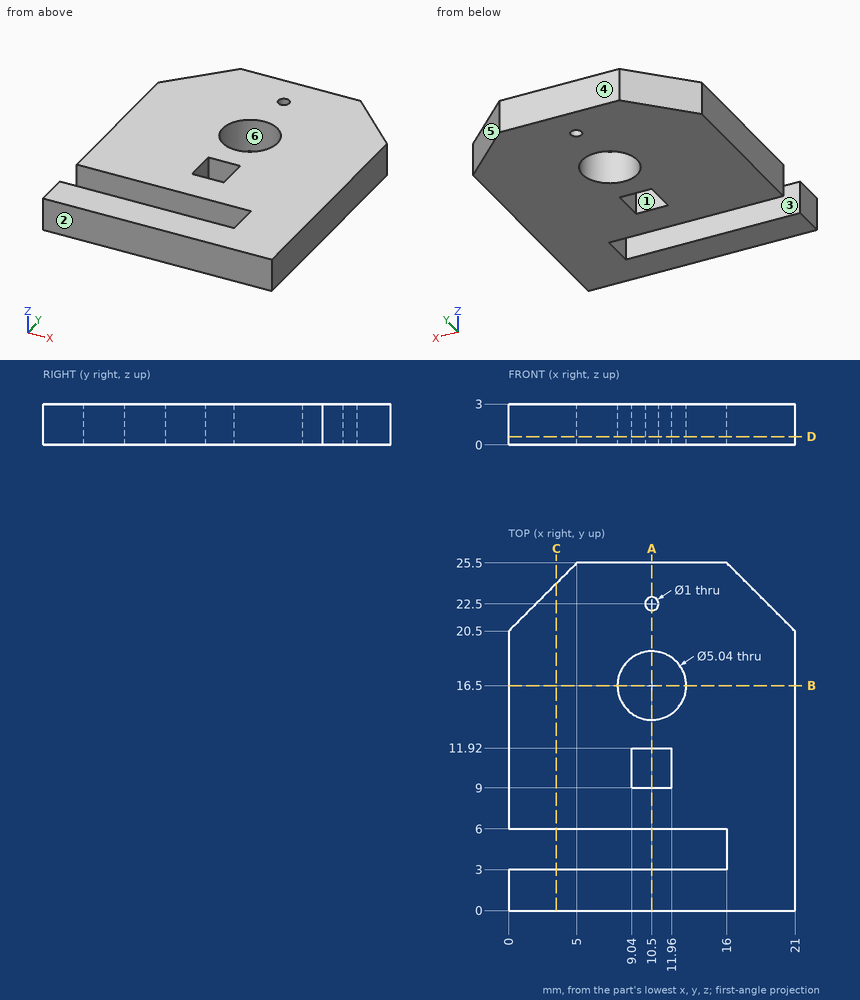
Print and shaded views of the part. All mm, measured from the part's lowest x, y and z. A direction names the side the tool comes from. Coordinates: 2 decimals unless noted, no trailing zeros. Order: outer loops, then holes, each group sorted by start corner. A loop starts at its lowest first (then second) coordinate and runs counter-clockwise, first axis right, second up.
Item 1: Saw through at D-D on z = 0.6. List the corners of the cut face in (x, y).
Filled in:
outline: (0, 0) - (21, 0) - (21, 20.5) - (16, 25.5) - (5, 25.5) - (0, 20.5) - (0, 6) - (16, 6) - (16, 3) - (0, 3) - close; hole circle Ø5.04 at (10.5, 16.5); hole (9.04, 9) - (11.96, 9) - (11.96, 11.92) - (9.04, 11.92) - close; hole circle Ø1 at (10.5, 22.5)
Item 2: Drill centre lines: L1, parallel to Y at x = 10.5, z = 1.95; L2, parallel to Y at x = 12.5, z = 0.55; L3, parallel to Y at x = 11.75, z = 0.4. Where is each one in solid material? Low to high.
Filled in:
L1: y = 0 to 3, 6 to 9, 11.92 to 13.98, 19.02 to 22, 23 to 25.5
L2: y = 0 to 3, 6 to 14.97, 18.03 to 25.5
L3: y = 0 to 3, 6 to 9, 11.92 to 14.31, 18.69 to 25.5
Item 3: Drop a flat-ended pin along its axis: pin 1 Ø0.9 at (y, z) = (4.5, 1) entering from -X. Give the stop position or say it passes through.
Filled in:
pin 1: stops at x = 16
Item 4: Saw through at B-B on y = 16.5. List the corners of the cut face in (x, z), then the cut area to 3 significant figures.
Filled in:
outline: (0, 0) - (7.98, 0) - (7.98, 3) - (0, 3) - close; (13.02, 0) - (21, 0) - (21, 3) - (13.02, 3) - close
area: 47.9 mm2
Item 5: Mould opens along X. For the marked faces 4, 5 and 6 say: released by +X, released by -X, zero draft, split by the parting line, or undercut.
Filled in:
face 4: zero draft
face 5: released by +X
face 6: undercut
Item 6: Saw through at C-C on x = 3.5. List the corners of the cut face in (y, z).
Filled in:
outline: (0, 0) - (3, 0) - (3, 3) - (0, 3) - close; (6, 0) - (24, 0) - (24, 3) - (6, 3) - close
Item 7: Saw through at A-A on x = 10.5. List the corners of the cut face in (y, z).
Filled in:
outline: (0, 0) - (3, 0) - (3, 3) - (0, 3) - close; (6, 0) - (9, 0) - (9, 3) - (6, 3) - close; (11.92, 0) - (13.98, 0) - (13.98, 3) - (11.92, 3) - close; (19.02, 0) - (22, 0) - (22, 3) - (19.02, 3) - close; (23, 0) - (25.5, 0) - (25.5, 3) - (23, 3) - close
Item 8: Tool access for the marked faces 1, 2 and 3: list every direction of +Z, -Z, +X, -X, +Y, -Y with a clear straight run to the whole face (end or side of a thin tool).
Filled in:
face 1: +Z, -Z
face 2: +Z, -Z, +X, -X, -Y
face 3: +Z, -Z, -X
